Check sheet for the modelled part. Datum: model origin and axes. Units: mm. A direction names the side the tool comes from. Coordinates: 2 decimals unless noted, no trailing zeros. Write each loop counter-clockwise with the first axis right and the second up, starting at its lowest first coordinate (ties: lowest second). Pieces come first, ordered by that corner, then holes. Notation, with made-up numbers: (42.25, 39) - (86.25, 39) arc R19 ccw to (86.25, 58) - close; hole circle Ø11 at (47, -26). An arc over 180 degrees is marked (long way). Use one line per item in the form item = value. Start each with the question number.
1. Cross-section at A-A on x = -7. Record the boundary of the cut face in (y, z).
2. Go/stop test with a flat-tipped pin: pin 1 Ø4 at (x, y) = (-28.49, -20.62) entering from +Z. Record where the tip stops, or that it passes through.
3. Cross-section at C-C on y = -22. Record the boundary of the cut face in (x, z), then the cut area to 3 significant figures.
4. Tool access check on faces 1 (the face through (-31.662, -20.764, 11.193)), 2 (the face through (-13.717, -12.522, 49.375)). Record the directions out of +Z, -Z, +X, -X, +Y, -Y that give a thin tool (end or side, any length) a straight path to the whole face; none if there is none.
5. Cross-section at B-B on z = 34. Record the boundary of the cut face in (x, y), then the cut area to 3 significant figures.
6. Scan lines: line 1 along Z through (x, y) = (-11, -16.5); line 2 along X through (y, z) = (-18, 17); line 3 along Z through (x, y) = (-15, -21.75). Record each from-to range of solid material in increasing order.
7. Draft check along Z on faces 3 (the face through (-16.969, -12.522, 17.934)), 4 (the face through (-19, 0, 18)), 5 (the face through (-29, -21, 17.632)). Enter one of: +Z half, -Z half, draft (parallel to the pull), parting line (faces both ways), or undercut.
8. Cross-section at D-D on z = 8.5. Give the number of separate pieces and of enclosed holes in the cut face, then the cut area to 3 significant figures.
```python
from build123d import *

# Parameters (mm, degrees)
F0_R     = 12.7
F1_DEPTH = 25.4
F2_R     = 3.175
F3_DEPTH = 12.7


with BuildPart() as f1:
    # F0 (on Front) → F1 (new body)
    with BuildSketch(Plane.XZ):
        with BuildLine():
            Line((4.8346, 4.932279), (4.833907, 30.332279))
            ThreePointArc((4.833907, 30.332279), (-14.135108, 49.381587), (-33.2654, 30.494248))
            Line((-33.2654, 30.494248), (-33.2654, 30.169272))
            Line((-33.2654, 30.169272), (-33.2654, 4.932279))
            Line((-33.2654, 4.932279), (4.8346, 4.932279))
        make_face()
        with Locations((-14.216093, 30.33176)):
            Circle(F0_R, mode=Mode.SUBTRACT)
        with BuildLine():
            Line((-33.2654, 30.169272), (-33.2654, 30.494248))
            ThreePointArc((-33.2654, 30.494248), (-33.266093, 30.33176), (-33.2654, 30.169272))
        make_face()
    extrude(amount=F1_DEPTH)

    # F2 (on face) → F3 (cut)
    with BuildSketch(Plane(origin=(0, 0, 4.932279), x_dir=(1, 0, 0), z_dir=(0, 0, -1))):
        with Locations((-28.4902, 20.6248)):
            Circle(F2_R)
        with Locations((0.0594, 20.6248)):
            Circle(F2_R)
    extrude(amount=-F3_DEPTH, mode=Mode.SUBTRACT)


solid = f1.part
```
Final values:
q1.outline = (-25.4, 4.93) - (0, 4.93) - (0, 19.88) - (-25.4, 19.88) - close; (-25.4, 40.78) - (0, 40.78) - (0, 47.96) - (-25.4, 47.96) - close
q2.pin_1 = 44.9
q3.outline = (-33.27, 4.93) - (-31.35, 4.93) - (-31.35, 17.63) - (-25.63, 17.63) - (-25.63, 4.93) - (-2.8, 4.93) - (-2.8, 17.63) - (2.92, 17.63) - (2.92, 4.93) - (4.83, 4.93) - (4.83, 30.33) arc R19.05 ccw to (-33.27, 30.49) arc R19.05 ccw to (-33.27, 30.17) - close; hole circle Ø25.4 at (-14.22, 30.33)
q3.area = 886 mm²
q4.face_1 = -Z
q4.face_2 = +Z, +Y, -Y
q5.outline = (-32.91, -25.4) - (-26.37, -25.4) - (-26.37, 0) - (-32.91, 0) - close; (-2.06, -25.4) - (4.48, -25.4) - (4.48, 0) - (-2.06, 0) - close
q5.area = 332 mm²
q6.line_1 = 4.93 to 18.05, 42.62 to 49.11
q6.line_2 = -33.27 to -30.28, -26.7 to -1.73, 1.85 to 4.83
q6.line_3 = 4.93 to 17.66, 43.01 to 49.37
q7.face_3 = undercut
q7.face_4 = draft
q7.face_5 = -Z half
q8.separate_pieces = 1
q8.enclosed_holes = 2
q8.area = 904 mm²
